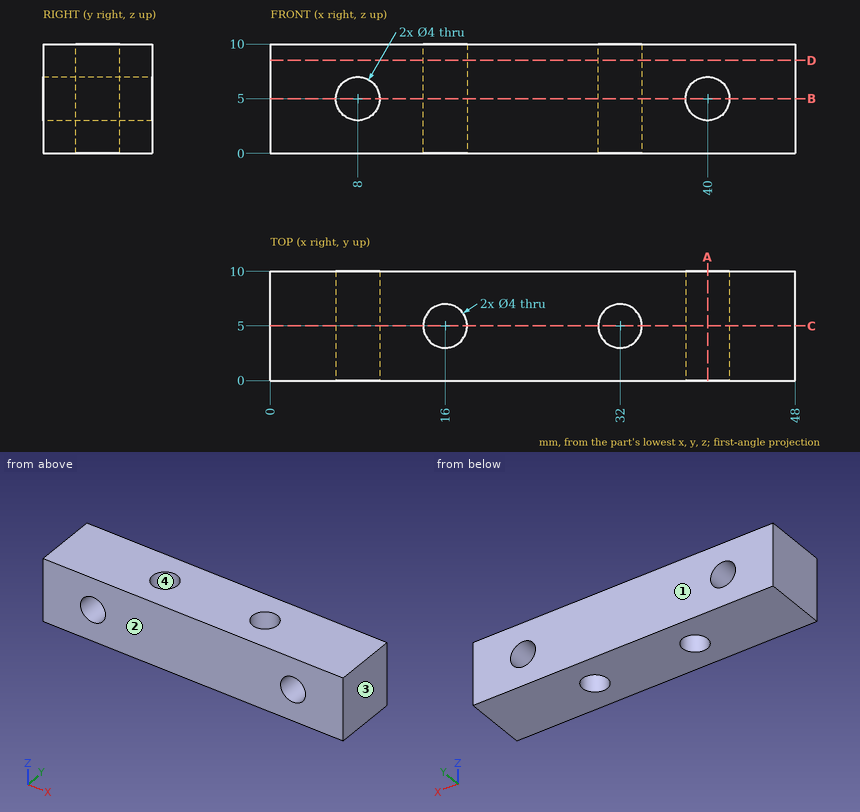
Source: three-view drawing plus pictorial views. Frame: mm from the lowest corner of the part. Coordinates: 2 decimals unless noted, no trailing zeros. Order: outer loops, then holes, each group sorted by start corner. A loop starts at its lowest first (then second) coordinate and runs counter-clockwise, first axis right, second up. Notation, with made-up numbers: M 53.25,78 L 75.25,78 A26 cw 75.25,100 Z; hole C -4,25 d2. An arc over 180 degrees is marked long. Write each question's results on one line, items separated by ' | '. Start each with the question number.
1. Draft query along Y for the marked faces 1, 2, 3 and 4. Return one class per face: +Y half, -Y half, draft (parallel to the pull), parting line (faces both ways), or undercut.
2. Material intervals for L1, parallel to X at y = 2.5, z = 5; L2, parallel to Y at x = 32, z = 6.5; L3, parallel to X at y = 6, z = 2.5, sorted ascending.
3. Section C-C, the plane y = 5. Return the cut outline in (x, z), then the cut area to 3 significant figures.
4. Section A-A, the plane x = 40. Return the cut outline in (y, z).
5. Section D-D, the plane z = 8.5. Return the cut outline in (x, y), then the cut area to 3 significant figures.
6. Section B-B, the plane z = 5. Return the cut outline in (x, y).
Solution:
1) face 1: +Y half | face 2: -Y half | face 3: draft | face 4: undercut
2) L1: 0 to 6, 10 to 38, 42 to 48 | L2: 0 to 3, 7 to 10 | L3: 0 to 14.27, 17.73 to 30.27, 33.73 to 48
3) outline: M 0,0 L 14,0 L 14,10 L 0,10 Z; M 18,0 L 30,0 L 30,10 L 18,10 Z; M 34,0 L 48,0 L 48,10 L 34,10 Z; hole C 8,5 d4; hole C 40,5 d4 | area: 375 mm²
4) outline: M 0,0 L 10,0 L 10,3 L 0,3 Z; M 0,7 L 10,7 L 10,10 L 0,10 Z
5) outline: M 0,0 L 48,0 L 48,10 L 0,10 Z; hole C 16,5 d4; hole C 32,5 d4 | area: 455 mm²
6) outline: M 0,0 L 6,0 L 6,10 L 0,10 Z; M 10,0 L 38,0 L 38,10 L 10,10 Z; M 42,0 L 48,0 L 48,10 L 42,10 Z; hole C 16,5 d4; hole C 32,5 d4
